Here's how the part is built. I have some questions about the finished solid (model axes, mm). Face numbers are marked on the shaded views. A direction names the side the tool comes from. Round coordinates to 2 decimals unless told otherwise and drop trailing zeros. Order: outer loops, then holes, each group sorted by start corner. A loop starts at its lowest first (then second) coordinate and runs counter-clockwise, first axis right, second up. Notation, with made-up numbers: (77, 8.5) -> (125, 8.5) arc R20 ccw to (125, 14.5) -> close; hole circle Ø10 at (51, 42.25). An arc over 180 degrees is marked (long way). One line per item, written item: value.
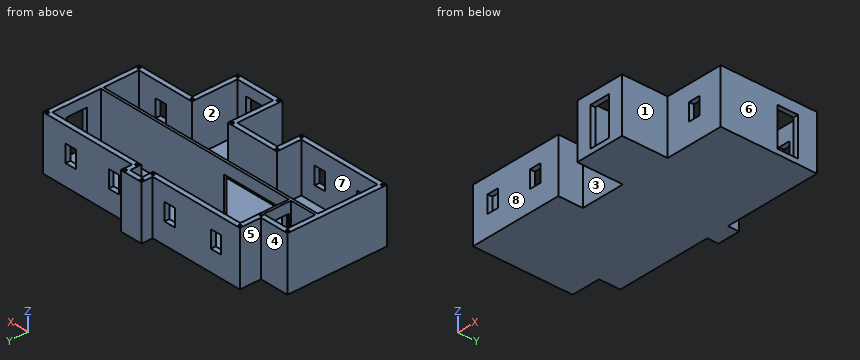
```python
from build123d import *

# Parameters (mm, degrees)
F0_R      = 0.6477
F0_R_2    = 0.6441405576
F0_W      = 1.27
F0_H      = 14.2598937347
F2_DEPTH  = 25.4
F12_DEPTH = 2.54
F4_W      = 5.8928
F4_H      = 8.9408
F3_W      = 5.8928
F3_H      = 8.9408
F13_DEPTH = 25.4
F6_W      = 5.8928
F6_H      = 8.9408
F5_W      = 10.5937230855
F5_H      = 19.9419036508
F7_W      = 5.8928
F7_H      = 8.9408
F14_DEPTH = 12.7
F10_W     = 10.5918
F10_H     = 19.939
F15_DEPTH = 12.7
F9_W      = 10.5918
F9_H      = 19.939
F16_DEPTH = 25.4
F8_W      = 32.9645648599
F8_H      = 19.3392261863
F17_DEPTH = 12.7


# Not quite as in the source:
# - the program builds the solid bodies; features that only make, move or delete a surface that nothing else refers to are left out


with BuildPart() as f2:
    # F0 (on Top) → F2 (new body)
    with BuildSketch(Plane.XY):
        Polygon((-45.4049956864, 2.54), (-47.9449956864, 2.54), (-47.9449956864, 0), (-47.9449956864, -8.4182334522), (-60.4807920754, -8.4182334522), (-63.0207920754, -8.4182334522), (-63.0207920754, -10.9582334522), (-63.0207920754, -57.4975824572), (-63.0207920754, -60.0375824572), (-60.4807920754, -60.0375824572), (-16.9454139954, -60.0375824572), (-14.4054139954, -60.0375824572), (-14.4054139954, -57.4975824572), (-14.4054139954, -47.3375824572), (8.416604454, -47.3375824572), (8.416604454, -68.4223124651), (8.416604454, -70.9623124651), (10.956604454, -70.9623124651), (31.4210504293, -70.9623124651), (33.9610504293, -70.9623124651), (33.9610504293, -68.4223124651), (33.9610504293, -47.3375824572), (61.6818144917, -47.3375824572), (64.2218144917, -47.3375824572), (64.2218144917, -44.7975824572), (64.2218144917, 0), (64.2218144917, 2.54), (61.6818144917, 2.54), (13.496604454, 2.54), (13.496604454, 5.7937128431), (13.496604454, 8.3337128431), (10.956604454, 8.3337128431), (4.2076310147, 8.3337128431), (1.6676310147, 8.3337128431), (1.6676310147, 5.7937128431), (1.6676310147, 2.54), align=None)
        with Locations((-61.7507920754, -58.7675824572)):
            Circle(F0_R, mode=Mode.SUBTRACT)
        with Locations((-15.6754139954, -58.7675824572)):
            Circle(F0_R, mode=Mode.SUBTRACT)
        with Locations((-15.6754139954, -46.0675824572)):
            Circle(F0_R, mode=Mode.SUBTRACT)
        with Locations((9.686604454, -69.6923124651)):
            Circle(F0_R, mode=Mode.SUBTRACT)
        with Locations((32.6910504293, -69.6923124651)):
            Circle(F0_R, mode=Mode.SUBTRACT)
        with Locations((9.686604454, -46.0675824572)):
            Circle(F0_R, mode=Mode.SUBTRACT)
        with Locations((32.6910504293, -46.0675824572)):
            Circle(F0_R, mode=Mode.SUBTRACT)
        with Locations((62.9518144917, -46.0675824572)):
            Circle(F0_R, mode=Mode.SUBTRACT)
        with Locations((-61.7507920754, -9.6882334522)):
            Circle(F0_R, mode=Mode.SUBTRACT)
        with Locations((-46.6749956864, -9.6882334522)):
            Circle(F0_R, mode=Mode.SUBTRACT)
        with Locations((-46.6749956864, 1.27)):
            Circle(F0_R_2, mode=Mode.SUBTRACT)
        Polygon((10.956604454, -68.4223124651), (10.956604454, -47.3375824572), (10.956604454, -44.7975824572), (8.416604454, -44.7975824572), (-14.4054139954, -44.7975824572), (-16.9454139954, -44.7975824572), (-16.9454139954, -47.3375824572), (-16.9454139954, -57.4975824572), (-60.4807920754, -57.4975824572), (-60.4807920754, -26.4881271869), (-60.4807920754, -25.2181271869), (-60.4807920754, -10.9582334522), (-47.9449956864, -10.9582334522), (-46.6749956864, -10.9582334522), (-45.4049956864, -10.9582334522), (-45.4049956864, -8.4182334522), (-45.4049956864, 0), (1.6676310147, 0), (4.2076310147, 0), (4.2076310147, 2.54), (4.2076310147, 5.7937128431), (10.956604454, 5.7937128431), (10.956604454, 2.54), (10.956604454, 0), (13.496604454, 0), (61.6818144917, 0), (61.6818144917, -25.2181271869), (61.6818144917, -26.4881271869), (61.6818144917, -44.7975824572), (33.9610504293, -44.7975824572), (31.4210504293, -44.7975824572), (31.4210504293, -47.3375824572), (31.4210504293, -68.4223124651), align=None, mode=Mode.SUBTRACT)
        with Locations((2.9376310147, 1.27)):
            Circle(F0_R, mode=Mode.SUBTRACT)
        with Locations((12.226604454, 1.27)):
            Circle(F0_R, mode=Mode.SUBTRACT)
        with Locations((2.9376310147, 7.0637128431)):
            Circle(F0_R, mode=Mode.SUBTRACT)
        with Locations((12.226604454, 7.0637128431)):
            Circle(F0_R, mode=Mode.SUBTRACT)
        with Locations((62.9518144917, 1.27)):
            Circle(F0_R, mode=Mode.SUBTRACT)
        Polygon((-60.4807920754, -26.4881271869), (61.6818144917, -26.4881271869), (61.6818144917, -25.2181271869), (-45.4049956864, -25.2181271869), (-46.6749956864, -25.2181271869), (-60.4807920754, -25.2181271869), align=None)
        with Locations((-46.0399956864, -18.0881803195)):
            Rectangle(F0_W, F0_H)
    extrude(amount=F2_DEPTH)

    # F11 (on face) → F12 (join)
    with BuildSketch(Plane(origin=(0, 0, 0), x_dir=(1, 0, 0), z_dir=(0, 0, -1))):
        Polygon((13.496604454, -8.3337128431), (13.496604454, -2.54), (64.2218144917, -2.54), (64.2218144917, 47.3375824572), (33.9610504293, 47.3375824572), (33.9610504293, 70.9623124651), (8.416604454, 70.9623124651), (8.416604454, 47.3375824572), (-14.4054139954, 47.3375824572), (-14.4054139954, 60.0375824572), (-63.0207920754, 60.0375824572), (-63.0207920754, 8.4182334522), (-47.9449956864, 8.4182334522), (-47.9449956864, -2.54), (1.6676310147, -2.54), (1.6676310147, -8.3337128431), align=None)
    extrude(amount=F12_DEPTH)

    # F4 (on face) + F3 (on face) → F13 (cut)
    with BuildSketch(Plane.XZ):
        with Locations((48.364430666, 12.7)):
            Rectangle(F4_W, F4_H)
        with Locations((23.7640291452, 12.7)):
            Rectangle(F4_W, F4_H)
    with BuildSketch(Plane.XZ):
        with Locations((-7.994512096, 12.7)):
            Rectangle(F3_W, F3_H)
        with Locations((-34.4051830471, 12.7)):
            Rectangle(F3_W, F3_H)
    extrude(amount=-F13_DEPTH, mode=Mode.SUBTRACT)

    # F6 (on face) + F5 (on face) + F7 (on face) → F14 (cut)
    with BuildSketch(Plane.XZ.offset(47.3375824572)):
        with Locations((49.0914324605, 12.7)):
            Rectangle(F6_W, F6_H)
    with BuildSketch(Plane.XZ.offset(70.9623124651)):
        with Locations((21.1888274417, 9.9709518254)):
            Rectangle(F5_W, F5_H)
    with BuildSketch(Plane.XZ.offset(60.0375824572)):
        with Locations((-27.5427140296, 12.7)):
            Rectangle(F7_W, F7_H)
        with Locations((-51.7941080034, 12.7)):
            Rectangle(F7_W, F7_H)
    extrude(amount=-F14_DEPTH, mode=Mode.SUBTRACT)

    # F10 (on face) → F15 (cut)
    with BuildSketch(Plane.YZ.offset(-45.4049956864)):
        with Locations((-18.8149667105, 9.9695)):
            Rectangle(F10_W, F10_H)
    extrude(amount=-F15_DEPTH, mode=Mode.SUBTRACT)

    # F9 (on face) → F16 (cut)
    with BuildSketch(Plane(origin=(61.6818144917, 0, 0), x_dir=(0, -1, 0), z_dir=(-1, 0, 0))):
        with Locations((12.6090635934, 9.9695)):
            Rectangle(F9_W, F9_H)
    extrude(amount=-F16_DEPTH, mode=Mode.SUBTRACT)

    # F8 (on face) → F17 (cut)
    with BuildSketch(Plane.XZ.offset(26.4881271869)):
        with Locations((-24.977594614, 9.6696130931)):
            Rectangle(F8_W, F8_H)
    extrude(amount=-F17_DEPTH, mode=Mode.SUBTRACT)


solid = f2.part
```
Q1. Which directions (+Z, -Z, +X, -X, +Y, -Y) give clear straight access to the entire face, cutting with the end or side of a thin tool? Please do the marked faces 1, 2, 3 and 4.
Answers:
face 1: +Z, -Z, +X, -Y
face 2: +Z
face 3: +Z, -Z, -Y
face 4: +Z, -Z, -X, +Y
Q2. I want a section at B-B on x = 23.5. Write out the boundary of the cut face in (y, z), then the cut area to 3 significant figures.
Answers:
outline: (-70.96, -2.54) -> (2.54, -2.54) -> (2.54, 8.23) -> (0, 8.23) -> (0, 0) -> (-25.22, 0) -> (-25.22, 25.4) -> (-26.49, 25.4) -> (-26.49, 0) -> (-70.96, 0) -> close; (-70.96, 19.94) -> (-68.42, 19.94) -> (-68.42, 25.4) -> (-70.96, 25.4) -> close; (0, 17.17) -> (2.54, 17.17) -> (2.54, 25.4) -> (0, 25.4) -> close
area: 275 mm2
Q3. I want a section at D-D on z = 6. Give the number of separate pieces and of enclosed holes in the cut face, then the cut area to 3 significant figures.
Answers:
separate pieces: 2
enclosed holes: 16
area: 1,130 mm2
Q4. I want a section at A-A on x = -19.5. Write out the boundary of the cut face in (y, z).
Answers:
outline: (-60.04, -2.54) -> (2.54, -2.54) -> (2.54, 25.4) -> (0, 25.4) -> (0, 0) -> (-57.5, 0) -> (-57.5, 25.4) -> (-60.04, 25.4) -> close; (-26.49, 19.34) -> (-25.22, 19.34) -> (-25.22, 25.4) -> (-26.49, 25.4) -> close
Q5. I want a section at C-C on y = -62.5. Write out the boundary of the cut face in (x, z), then the cut area to 3 significant figures.
Answers:
outline: (8.42, -2.54) -> (33.96, -2.54) -> (33.96, 25.4) -> (31.42, 25.4) -> (31.42, 0) -> (10.96, 0) -> (10.96, 25.4) -> (8.42, 25.4) -> close
area: 194 mm2
Q6. If we mould it in two halves opening along X, with no side actions, what happens to the marked faces 5, 6, 7 and 8? For each: pulls with the +X half, pulls with the -X half, needs draft (parallel to the pull), parting line crosses it, or undercut.
Answers:
face 5: pulls with the -X half
face 6: pulls with the +X half
face 7: undercut
face 8: needs draft
Q7. I need wall thicknesses on line 1 along Y through (x, z) = (-30.5, 21.75); line 2 along X through (y, z) = (-23, 21.75) (3 decimals); line 3 along X through (y, z) = (-57, 3.5). Which ranges of each line are inside material? Lowest first, please.
Answers:
line 1: -60.04 to -57.5, -26.49 to -25.22, 0 to 2.54
line 2: -63.021 to -60.481, -46.675 to -45.405, 61.682 to 64.222
line 3: -63.02 to -60.48, -16.95 to -14.41, 8.42 to 10.96, 31.42 to 33.96
Q8. For P1, Ø0.8, axis at x = 2.94, y = 7.06, coming from the +Z side; P2, Ø2, axis at x = -0.5, z = 22.5, coming from the +Y side; P3, Ø3, axis at y = -58, z = 12.5, coming from the +X side, each with a flat end and sliding along its axis, tell me the tip position at first contact or that it passes through.
Answers:
P1: z = 0
P2: y = 2.54
P3: x = 33.96
